from build123d import *

# Parameters (mm, degrees)
SKETCH1_W                                    = 91.1352
SKETCH1_H                                    = 17.3863
BOSS_EXTRUDE1_DEPTH                          = 13.1826
SKETCH2_W                                    = 52.8828
SKETCH2_H                                    = 17.3863
CUT_EXTRUDE1_DEPTH                           = 7.239
CBORE_FOR_1_4_BINDING_HEAD_MACHINE_S_2_COUNT = 2
CBORE_FOR_1_4_BINDING_HEAD_MACHINE_S_2_PITCH = 72.009
SKETCH7_W                                    = 17.8181
SKETCH7_H                                    = 8.001
SKETCH7_W_2                                  = 18.3642
BOSS_EXTRUDE2_DEPTH                          = 7.9375


with BuildPart() as part:
    # Sketch1 → Boss-Extrude1 (new body)
    with BuildSketch(Plane.XY):
        with Locations((-45.5676, 8.69315)):
            Rectangle(SKETCH1_W, SKETCH1_H)
    extrude(amount=BOSS_EXTRUDE1_DEPTH)

    # Sketch2 → Cut-Extrude1 (cut)
    with BuildSketch(Plane.XY.offset(13.1826)):
        with Locations((-45.5676, 8.69315)):
            Rectangle(SKETCH2_W, SKETCH2_H)
    extrude(amount=-CUT_EXTRUDE1_DEPTH, mode=Mode.SUBTRACT)

    # Sketch6 → CBORE for 1/4 Binding Head Machine Screw1 (revolve, cut)
    with BuildSketch(Plane(origin=(-81.5721, 8.69315, 13.1826), x_dir=(0, -1, 0), z_dir=(1, 0, 0))):
        Polygon((0, 0), (0, 13.1826), (3.2639, 13.1826), (3.2639, 4.191), (7.14375, 4.191), (7.14375, 0.635), (7.77875, 0), align=None)
    cbore_for_1_4_binding_head_machine_screw = revolve(axis=Axis((-81.5721, 8.69315, 19.5326), (0, 0, -1)), mode=Mode.SUBTRACT)

    # CBORE for 1_4 Binding Head Machine S 2: CBORE for 1/4 Binding Head Machine Screw1 ×2
    with Locations(*[(i * CBORE_FOR_1_4_BINDING_HEAD_MACHINE_S_2_PITCH, 0, 0) for i in range(1, CBORE_FOR_1_4_BINDING_HEAD_MACHINE_S_2_COUNT)]):
        add(cbore_for_1_4_binding_head_machine_screw, mode=Mode.SUBTRACT)

    # Sketch7 → Boss-Extrude2 (add)
    with BuildSketch(Plane.XY.offset(5.9436)):
        with Locations((-56.52135, 13.3858)):
            Rectangle(SKETCH7_W, SKETCH7_H)
        with Locations((-34.8742, 13.3858)):
            Rectangle(SKETCH7_W_2, SKETCH7_H)
    extrude(amount=BOSS_EXTRUDE2_DEPTH)


solid = part.part
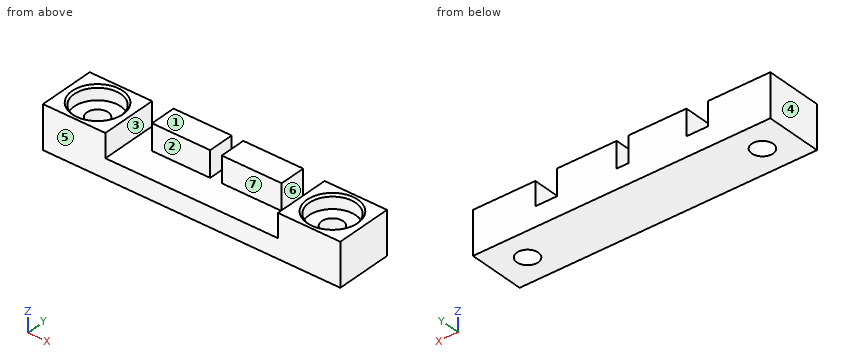
Here's how the part is built. I have some questions about the finished solid (model axes, mm). Face numbers are marked on the shaded views. A direction names the side the tool comes from. Give positions to 0.01 mm unless a question says otherwise; leave off trailing zeros. Order: outer loops, then holes, each group sorted by start corner. A loop starts at its lowest first (then second) coordinate and runs counter-clockwise, first axis right, second up. Notation, with made-up numbers: M 42,-30.75 L 63,-30.75 A19 cw 63,-16.75 Z; hole C 6,86.25 d10. An arc over 180 degrees is marked long. Answer as a JSON object with one key per item and string values. Group by question number.
1) Suppose I cut it at B-B, the plane x = -54. Write out the boundary of the cut face in (y, z).
2) Please list where these lines run through material, in increasing order: L1, parallel to X at y = 8.75, z = 2.75; L2, parallel to X at y = 2.5, z = 10; L3, parallel to X at y = 16.25, z = 7.75. Write a range as [from, to].
3) I'm going to push flat-ended pins straight in: pin 1 Ø1.5 at (x, y) = (-43, 2) entering from +Z; pin 2 Ø8.5 at (x, y) = (-9.56, 8.69) entering from +Z. Where does each tip first touch, or does it pass through?
4) Suppose I cut it at A-A, the plane z = 10.5. Write out the boundary of the cut face in (x, y), plus the area to 3 significant figures.
5) Suppose I cut it at C-C, the plane z = 5. Write out the boundary of the cut face in (x, y).
6) On a 3-axis mill with a long thin cutter (end or side, diameter ignored), from which of +Z, -Z, +X, -X, +Y, -Y can I reach the whole of each face in a straight line? I mean the marked faces 1, 2 and 3. Say none if no direction works.
7) We'd pull the mould along X, two halves only. Please class the marked faces 4, 5, 6 and 7: pulls with the +X half, pulls with the -X half, needs draft (parallel to the pull), parting line crosses it, or undercut.
Results found:
{
 "1": {"outline": "M 0,0 L 17.39,0 L 17.39,13.88 L 9.39,13.88 L 9.39,5.94 L 0,5.94 Z"},
 "2": {"L1": "[-91.14, -84.84], [-78.31, -12.83], [-6.3, 0]", "L2": "[-91.14, -85.13], [-78.01, -72.01], [-19.13, -13.12], [-6, 0]", "L3": "[-91.14, -72.01], [-65.43, -47.61], [-44.06, -25.69], [-19.13, 0]"},
 "3": {"pin 1": "z = 5.94", "pin 2": "z = 8.99"},
 "4": {"outline": "M -91.14,0 L -72.01,0 L -72.01,17.39 L -91.14,17.39 Z; M -65.43,9.39 L -47.61,9.39 L -47.61,17.39 L -65.43,17.39 Z; M -44.06,9.39 L -25.69,9.39 L -25.69,17.39 L -44.06,17.39 Z; M -19.13,0 L 0,0 L 0,17.39 L -19.13,17.39 Z; hole C -81.57,8.69 d14.29; hole C -9.56,8.69 d14.29", "area": "634 mm²"},
 "5": {"outline": "M -91.14,0 L 0,0 L 0,17.39 L -91.14,17.39 Z; hole C -81.57,8.69 d6.53; hole C -9.56,8.69 d6.53"},
 "6": {"face 1": "+Z, +X, -X, +Y, -Y", "face 2": "+Z, -Y", "face 3": "+Z, +Y, -Y"},
 "7": {"face 4": "pulls with the -X half", "face 5": "needs draft", "face 6": "undercut", "face 7": "undercut"}
}
